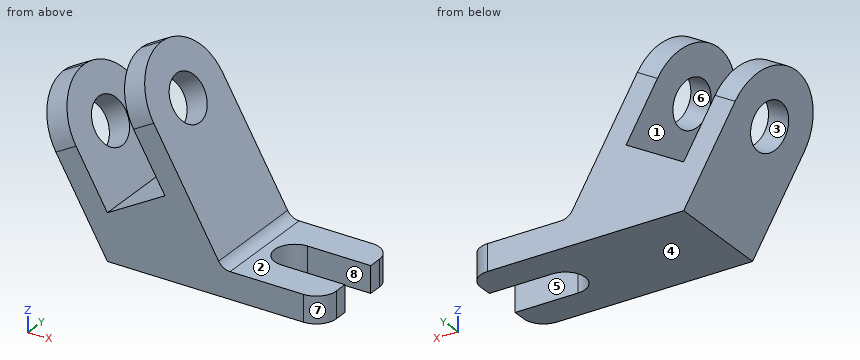
```python
from build123d import *

# Parameters (mm, degrees)
F1_DEPTH = 25.4
F3_DEPTH = 12.701
F5_D     = 22.225
F6_R     = 25.39999
F7_R     = 9.525


# Not quite as in the source:
# - a fillet or chamfer is up to 0.001 mm smaller than in the source, because OpenCascade refuses the exact size


with BuildPart() as f1:
    # F0 (on Front) → F1 (new body, symmetric)
    with BuildSketch(Plane.XZ):
        with BuildLine():
            Line((-37.30625, 64.6163204399), (0, 0))
            Line((0, 0), (103.1875, 0))
            Line((103.1875, 0), (103.1875, 12.7))
            Line((103.1875, 12.7), (58.6587873497, 12.7))
            ThreePointArc((58.6587873497, 12.7), (55.4837873497, 13.550738686), (53.1595260356, 15.875))
            Line((53.1595260356, 15.875), (9.4374711693, 91.6038204399))
            Line((9.4374711693, 91.6038204399), (-0.1862361303, 86.0475704399))
            Line((-0.1862361303, 86.0475704399), (27.4963065702, 38.1))
            Line((27.4963065702, 38.1), (0, 22.225))
            Line((0, 22.225), (-27.6825427004, 70.1725704399))
            Line((-27.6825427004, 70.1725704399), (-37.30625, 64.6163204399))
        make_face()
    extrude(amount=F1_DEPTH, both=True)

    # F2 (on face) → F3 (cut, through all)
    with BuildSketch(Plane.XY.offset(12.7)):
        with BuildLine():
            Line((103.1875, 9.525), (73.025, 9.525))
            ThreePointArc((73.025, 9.525), (63.5, 0), (73.025, -9.525))
            Line((73.025, -9.525), (103.1875, -9.525))
            Line((103.1875, -9.525), (103.1875, 9.525))
        make_face()
    extrude(amount=-F3_DEPTH, mode=Mode.SUBTRACT)

    # F5 (through all)
    with Locations(Plane(origin=(46.7437211693, 0, 26.9875), x_dir=(0, 1, 0), z_dir=(0.8660254038, 0, 0.5))):
        with Locations((0, 49.2125)):
            Hole(F5_D / 2)

    # F6 (radius 25.4 in the source; OpenCascade refuses exactly that, so slightly less here)
    f6_edges = [f1.edges().sort_by_distance(p)[0] for p in [
        (-32.494396, 25.4, 67.394445),
        (4.625618, 25.4, 88.825695),
        (-32.494396, -25.4, 67.394445),
        (4.625618, -25.4, 88.825695),
    ]]
    fillet(f6_edges, radius=F6_R)

    # F7
    f7_edges = [f1.edges().sort_by_distance(p)[0] for p in [
        (103.1875, 25.4, 6.35),
        (103.1875, -25.4, 6.35),
    ]]
    fillet(f7_edges, radius=F7_R)


solid = f1.part
```
The listing builds one solid part. Answer for the finished solid, in the listing's coordinates (mm). Face numbers are marked on the shaded views. A direction names the side the tool comes from. Give positions to 0.01 mm unless a question says otherwise; leave off trailing zeros. Order: outer loops, then holes, each group sorted by start corner. A loop starts at its lowest first (then second) coordinate and runs counter-clockwise, first axis right, second up. Notation, with made-up numbers: (59.5, 18.25) - (75.5, 18.25) arc R30 cw to (75.5, 48.25) - close; hole circle Ø1 at (20.25, 46). An arc over 180 degrees is marked (long way). Use one line per item in the form item = value. Start each with the question number.
(1) For the marked faces 1, 2, 3, 4 and 5, determine the directions among +Z, -Z, +X, -X, +Y, -Y from which every point of the face is accessible in a straight line to the end or side of a thin tool.
(2) Consider line 1 (Z direction, x = 83, y = 21.5); line 2 (X direction, y = -7, z = 61.5); line 3 (X direction, y = -15, z = 36.5). Determine where each line is inside the solid, lowest interval first. Write a range as from..to.
(3) A cutting plane is placed at D-D, the plane x = 61. Write down the section's boundary in (y, z).
(4) The mould has two halves that part along X. Classify the marked faces 6, 7 and 8: released by +X, released by -X, zero draft, split by the parting line, or undercut.
(5) A cutting plane is placed at C-C, the plane z = 51. State how many separate pieces and enclosed holes the cut face has, then the cut area to 3 significant figures.
(6) A cutting plane is placed at B-B, the plane y = 3.5. Write down the section's boundary in (x, z) (3 decimals).
(7) A cutting plane is placed at A-A, the plane x = 91. Write down the section's boundary in (y, z) (3 decimals).
(8) Flat-ended cylindrical pins translate along their axes: pin 1 Ø13.5 at (x, y) = (79, 4.5) entering from +Z; pin 2 Ø10 at (x, y) = (22.5, -18) entering from +Z; pin 3 Ø5 at (y, z) = (-7, 33.5) entering from -X; pin 4 Ø6 at (x, y) = (60, -18.5) entering from -Z. Find the tip coordinate at first contact, or state that the pin passes through.
Ans:
q1.face_1 = +Y, -Y
q1.face_2 = +Z, +X, +Y, -Y
q1.face_3 = none
q1.face_4 = -Z, +X, -X, +Y, -Y
q1.face_5 = +Z, -Z, +X
q2.line_1 = 0..12.7
q2.line_2 = -35.51..-22.68, 25.36..26.82
q2.line_3 = -21.07..-8.24, 24.73..41.25
q3.outline = (-25.4, 0) - (25.4, 0) - (25.4, 12.7) - (-25.4, 12.7) - close
q4.face_6 = undercut
q4.face_7 = released by +X
q4.face_8 = zero draft
q5.separate_pieces = 3
q5.enclosed_holes = 0
q5.area = 1,060 mm^2
q6.outline = (-37.185, 64.406) - (-29.88, 51.753) - (-20.256, 57.309) - (-27.561, 69.963) - close; (-19.333, 33.485) - (0, 0) - (64.166, 0) - (64.166, 12.7) - (58.659, 12.7) arc R6.35 cw to (53.16, 15.875) - (27.411, 60.473) - (17.787, 54.917) - (27.496, 38.1) - (0, 22.225) - (-9.709, 39.042) - close; (-0.065, 85.838) - (7.24, 73.184) - (16.864, 78.741) - (9.559, 91.394) - close
q7.outline = (-25.4, 0) - (-9.525, 0) - (-9.525, 12.7) - (-25.4, 12.7) - close; (9.525, 0) - (25.4, 0) - (25.4, 12.7) - (9.525, 12.7) - close
q8.pin_1 = 12.7
q8.pin_2 = 77.64
q8.pin_3 = -20.69
q8.pin_4 = 0
